The model under review builds one solid part; all positions refer to its coordinate system, in mm. A direction names the side the tool comes from. Coordinates: 2 decimals unless noted, no trailing zeros. Write each loop counter-clockwise with the first axis right and the second up, starting at its lowest first coordinate (ties: lowest second). Pieces come first, ordered by that corner, then holes. Notation, with made-up numbers: (83, 60) - (95, 60) arc R12 ccw to (95, 83) - close; hole circle Ø3 at (-15.5, 24.25). An arc over 180 degrees is marked (long way). Return JSON: item names as keys, results as strings. Group by question number.
(1) For pin 1 Ø4 at (x, y) = (-20, 30) entering from -Z; pin 2 Ø1.5 at (x, y) = (-19, 30.5) entering from +Z; pin 3 Ø3 at (x, z) = (-16, 1.5) entering from -Y, all flat-tipped, find the tip position at first contact; note any pin that passes through.
(2) We need section B-B on x = -27. State the section outline as (y, z) points, then the cut area to 3 significant figures.
(3) To check wall thickness, follow L1, parallel to Z at x = -12, y = 28; L2, parallel to X at y = 4, z = 0.25; L3, parallel to Y at x = -15, z = -3. State the ranges of each line that lie inside material, in increasing order. Write a range as from..to.
(4) Tool access review of faces 1 (the face through (-12, 32, 0)), 2 (the face through (0, 13, 1.901)), 3 (the face through (-15, 29, -4.9)), 4 (the face through (0.186, 13.311, -4.896)): name each direction out of +Z, -Z, +X, -X, +Y, -Y from which nothing blocks a thin tool from reaching the whole face with its end or side.
(5) We need section D-D on z = 0.05. State the section outline as (x, y) points, then the cut area to 3 significant figures.
(6) We need section A-A on z = -4. State the section outline as (x, y) points, then the cut area to 3 significant figures.
(7) Draft analysis for pull direction X (two halves, no side actions). For faces 5 (the face through (-2.05, 13, 3)), 6 (the face through (-15, 29, 5)), 7 (the face through (-30, 29, 0)), 8 (the face through (2.05, 13, 3)), state which applies: released by +X, released by -X, zero draft, split by the parting line, or undercut.
(8) We need section C-C on y = 15.5. State the section outline as (x, z) points.
```python
from build123d import *

# Parameters (mm, degrees)
SKETCH1_R           = 4.9
BOSS_EXTRUDE1_DEPTH = 27
CUT_EXTRUDE1_START  = -28
CUT_EXTRUDE1_DEPTH  = 28
BOSS_EXTRUDE2_DEPTH = 5


with BuildPart() as part:
    # Sketch1 → Boss-Extrude1 (new body)
    with BuildSketch(Plane(origin=(0, 0, 0), x_dir=(1, 0, 0), z_dir=(0, 1, 0))):
        with Locations(Location((0, 0, 0), (0, 0, 270))):
            Circle(SKETCH1_R)
    extrude(amount=BOSS_EXTRUDE1_DEPTH)

    # Sketch3 → Cut-Extrude1 (cut)
    with BuildSketch(Plane(origin=(0, 27, 0), x_dir=(1, 0, 0), z_dir=(0, 1, 0)).offset(CUT_EXTRUDE1_START)):
        with BuildLine():
            Line((-2.05, -4.450561762), (-2.05, -1.900561762))
            Line((-2.05, -1.900561762), (2.05, -1.900561762))
            Line((2.05, -1.900561762), (2.05, -4.450561762))
            ThreePointArc((2.05, -4.450561762), (0, -4.9), (-2.05, -4.450561762))
        make_face()
    extrude(amount=CUT_EXTRUDE1_DEPTH, mode=Mode.SUBTRACT)

    # Sketch2 → Boss-Extrude2 (add)
    with BuildSketch(Plane(origin=(0, 27, 0), x_dir=(1, 0, 0), z_dir=(0, 1, 0))):
        with BuildLine():
            Line((0, 4.9), (-30, 4.9))
            Line((-30, 4.9), (-30, -5))
            Line((-30, -5), (0, -5))
            ThreePointArc((0, -5), (5.705336799, -0.05), (0, 4.9))
        make_face()
    extrude(amount=BOSS_EXTRUDE2_DEPTH)


solid = part.part
```
Ans:
{
 "1": {"pin 1": "z = -4.9", "pin 2": "z = 5", "pin 3": "y = 27"},
 "2": {"outline": "(27, -4.9) - (32, -4.9) - (32, 5) - (27, 5) - close", "area": "49.5 mm²"},
 "3": {"L1": "-4.9..5", "L2": "-4.89..4.89", "L3": "27..32"},
 "4": {"face 1": "+Z, -Z, +X, -X, +Y", "face 2": "+Z, -Y", "face 3": "-Z, -X, +Y, -Y", "face 4": "-Y"},
 "5": {"outline": "(-30, 27) - (-4.9, 27) - (-4.9, 0) - (4.9, 0) - (4.9, 27) - (5.71, 27) - (5.71, 32) - (-30, 32) - close", "area": "443 mm²"},
 "6": {"outline": "(-30, 27) - (-2.83, 27) - (-2.83, 0) - (2.83, 0) - (2.83, 27) - (3.64, 27) - (3.64, 32) - (-30, 32) - close", "area": "321 mm²"},
 "7": {"face 5": "undercut", "face 6": "zero draft", "face 7": "released by -X", "face 8": "undercut"},
 "8": {"outline": "(-2.05, 1.9) - (-2.05, 4.45) arc R4.9 ccw (long way) to (2.05, 4.45) - (2.05, 1.9) - close"}
}
